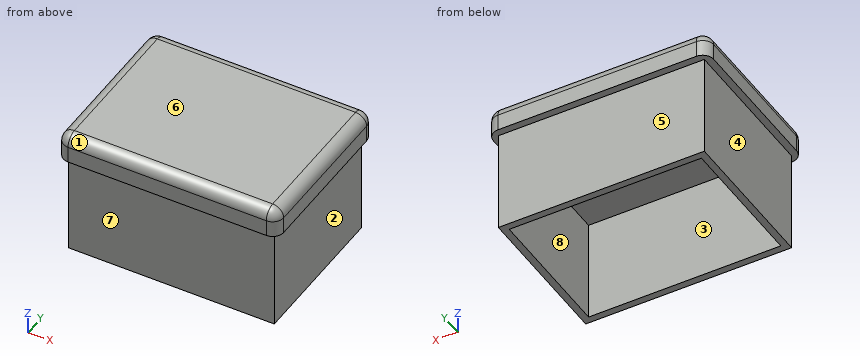
from build123d import *

# Parameters (mm, degrees)
F0_W     = 101.6
F0_H     = 76.2
F1_DEPTH = 12.7
F2_R     = 5.08
F3_W     = 94.996
F3_H     = 69.596
F3_W_2   = 88.646
F3_H_2   = 63.246
F4_DEPTH = 47.625


with BuildPart() as f1:
    # F0 (on Top) → F1 (new body)
    with BuildSketch(Plane.XY):
        Rectangle(F0_W, F0_H)
    extrude(amount=F1_DEPTH)

    # F2
    f2_edges = [f1.edges().sort_by_distance(p)[0] for p in [
        (0, -38.1, 12.7),
        (-50.8, 0, 12.7),
        (0, 38.1, 12.7),
        (50.8, 0, 12.7),
        (50.8, -38.1, 6.35),
        (50.8, 38.1, 6.35),
        (-50.8, 38.1, 6.35),
        (-50.8, -38.1, 6.35),
    ]]
    fillet(f2_edges, radius=F2_R)

    # F3 (on face) → F4 (join)
    with BuildSketch(Plane(origin=(0, 0, 0), x_dir=(1, 0, 0), z_dir=(0, 0, -1))):
        Rectangle(F3_W, F3_H)
        Rectangle(F3_W_2, F3_H_2, mode=Mode.SUBTRACT)
    extrude(amount=F4_DEPTH)


solid = f1.part
Can you work these out from the model? Positions are in its coordinate system, mm. Face numbers are marked on the shaded views. A direction names the side the tool comes from. Coordinates: 2 decimals unless noted, no trailing zeros. Loops run counter-clockwise (first coordinate to the right, second up) from the corner with the lowest first, then second, coordinate; pieces in that order, holes last. Notation, with made-up numbers: M 88.5,80 L 94.5,80 A26 ccw 94.5,97 Z; hole C -28.5,38.5 d11. An arc over 180 degrees is marked long. Return JSON: item names as keys, results as strings. Group by question number.
Item 1: On a 3-axis mill with a long thin cutter (end or side, diameter ignored), from which of +Z, -Z, +X, -X, +Y, -Y can I reach the whole of each face in a straight line? I mean the marked faces 1, 2, 3, 4 and 5. Say none if no direction works.
Item 2: I'm going to push flat-ended pins straight in: pin 1 Ø14.5 at (y, z) = (0.5, -19) entering from +X; pin 2 Ø14.5 at (x, z) = (-21, -33) entering from -Y; pin 3 Ø23 at (x, y) = (3, 0) entering from -Z. Where does each tip first touch, or does it pass through?
Item 3: If I drill on L1, parallel to Y at x = 27, z = -37; L2, parallel to X at y = 0.5, z = -36; L3, parallel to Z at x = 29.5, y = 21.5, over which ranges is the centre line in solid material (lowest first)? Write a range as from..to.
Item 4: Thinking about a two-plate mould opening in Y: for the marked faces 6, 7 and 8, which applies, released by +Y, released by -Y, zero draft, split by the parting line, or undercut?
Item 5: Imagine slicing it at B-B (x = 4). Please give me the cut outline in (y, z) (3 decimals), and give its area (3 significant figures).
Item 6: Imagine slicing it at A-A (z = -13). Please give me the cut outline in (x, y), and give its area (3 significant figures).
Item 7: Imagine slicing it at C-C (y = 30). Please give me the cut outline in (x, z) (3 decimals), and give its area (3 significant figures).
Verdict:
{
 "1": {"face 1": "+Z, +X, -X, -Y", "face 2": "-Z, +X, +Y, -Y", "face 3": "-Z", "face 4": "-Z, -X, +Y, -Y", "face 5": "-Z, +X, -X, +Y"},
 "2": {"pin 1": "stops at x = 47.5", "pin 2": "stops at y = -34.8", "pin 3": "stops at z = 0"},
 "3": {"L1": "y = -34.8..-31.62, 31.62..34.8", "L2": "x = -47.5..-44.32, 44.32..47.5", "L3": "z = 0..12.7"},
 "4": {"face 6": "zero draft", "face 7": "released by -Y", "face 8": "undercut"},
 "5": {"outline": "M -38.1,0 L -34.798,0 L -34.798,-47.625 L -31.623,-47.625 L -31.623,0 L 31.623,0 L 31.623,-47.625 L 34.798,-47.625 L 34.798,0 L 38.1,0 L 38.1,7.62 A5.08 ccw 33.02,12.7 L -33.02,12.7 A5.08 ccw -38.1,7.62 Z", "area": "1,260 mm^2"},
 "6": {"outline": "M -47.5,-34.8 L 47.5,-34.8 L 47.5,34.8 L -47.5,34.8 Z; hole M -44.32,-31.62 L 44.32,-31.62 L 44.32,31.62 L -44.32,31.62 Z", "area": "1,000 mm^2"},
 "7": {"outline": "M -50.8,0 L -47.498,0 L -47.498,-47.625 L -44.323,-47.625 L -44.323,0 L 44.323,0 L 44.323,-47.625 L 47.498,-47.625 L 47.498,0 L 50.8,0 L 50.8,7.62 A5.08 ccw 45.72,12.7 L -45.72,12.7 A5.08 ccw -50.8,7.62 Z", "area": "1,580 mm^2"}
}
